Could you check a few things on this model? Use its own coordinates, in mm. Face numbers are marked on the shaded views. A direction names the side the tool comes from. Coordinates: 2 decimals unless noted, no trailing zeros. Order: outer loops, then holes, each group sorted by start corner. A loop starts at its lowest first (then second) coordinate and runs counter-clockwise, first axis right, second up. Notation, with made-up numbers: M -18,55 L 26,55 A16 cw 26,73 Z; hole C -9,78 d2. An arc over 180 degrees is marked long. One line per question, with ' | ' between items. Start each with the question number.
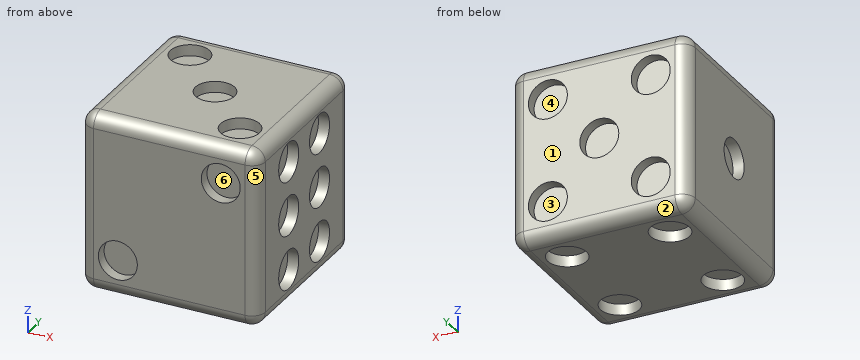
from build123d import *

# Parameters (mm, degrees)
F0_W      = 16
F0_H      = 16
F1_DEPTH  = 16
F2_R      = 1.75
F3_DEPTH  = 1
F4_R      = 1.75
F5_DEPTH  = 1
F6_R      = 1.75
F7_DEPTH  = 1
F8_R      = 1.75
F9_DEPTH  = 1
F10_R     = 1.75
F11_DEPTH = 1
F12_R     = 1.75
F13_DEPTH = 1
F14_R     = 1.2


with BuildPart() as f1:
    # F0 (on Top) → F1 (new body)
    with BuildSketch(Plane.XY):
        Rectangle(F0_W, F0_H)
    extrude(amount=F1_DEPTH)

    # F2 (on face) → F3 (cut)
    with BuildSketch(Plane.XY.offset(16)):
        with Locations((-4.618718, 4.618718)):
            Circle(F2_R)
        with Locations((4.618718, -4.618718)):
            Circle(F2_R)
        Circle(F2_R)
    extrude(amount=-F3_DEPTH, mode=Mode.SUBTRACT)

    # F4 (on face) → F5 (cut)
    with BuildSketch(Plane.XZ.offset(8)):
        with Locations((-4.618718, 3.381282)):
            Circle(F4_R)
        with Locations((4.618718, 12.618718)):
            Circle(F4_R)
    extrude(amount=-F5_DEPTH, mode=Mode.SUBTRACT)

    # F6 (on face) → F7 (cut)
    with BuildSketch(Plane(origin=(-8, 0, 0), x_dir=(0, -1, 0), z_dir=(-1, 0, 0))):
        with Locations((0, 8)):
            Circle(F6_R)
    extrude(amount=-F7_DEPTH, mode=Mode.SUBTRACT)

    # F8 (on face) → F9 (cut)
    with BuildSketch(Plane.YZ.offset(8)):
        with Locations((-2.7, 8)):
            Circle(F8_R)
        with Locations((2.7, 8)):
            Circle(F8_R)
        with Locations((2.7, 12.875)):
            Circle(F8_R)
        with Locations((2.7, 3.125)):
            Circle(F8_R)
        with Locations((-2.7, 3.125)):
            Circle(F8_R)
        with Locations((-2.7, 12.875)):
            Circle(F8_R)
    extrude(amount=-F9_DEPTH, mode=Mode.SUBTRACT)

    # F10 (on face) → F11 (cut)
    with BuildSketch(Plane(origin=(0, 8, 0), x_dir=(-1, 0, 0), z_dir=(0, 1, 0))):
        with Locations((0, 8)):
            Circle(F10_R)
        with Locations((-4.618718, 3.381282)):
            Circle(F10_R)
        with Locations((-4.618718, 12.618718)):
            Circle(F10_R)
        with Locations((4.618718, 12.618718)):
            Circle(F10_R)
        with Locations((4.618718, 3.381282)):
            Circle(F10_R)
    extrude(amount=-F11_DEPTH, mode=Mode.SUBTRACT)

    # F12 (on face) → F13 (cut)
    with BuildSketch(Plane(origin=(0, 0, 0), x_dir=(1, 0, 0), z_dir=(0, 0, -1))):
        with Locations((4.618718, -4.618718)):
            Circle(F12_R)
        with Locations((-4.618718, -4.618718)):
            Circle(F12_R)
        with Locations((-4.618718, 4.618718)):
            Circle(F12_R)
        with Locations((4.618718, 4.618718)):
            Circle(F12_R)
    extrude(amount=-F13_DEPTH, mode=Mode.SUBTRACT)

    # F14
    f14_edges = [f1.edges().sort_by_distance(p)[0] for p in [
        (0, 8, 16),
        (-8, 0, 16),
        (-8, 8, 8),
        (-8, -8, 8),
        (0, -8, 16),
        (8, -8, 8),
        (8, 0, 0),
        (8, 8, 8),
        (0, 8, 0),
        (-8, 0, 0),
        (0, -8, 0),
        (8, 0, 16),
    ]]
    fillet(f14_edges, radius=F14_R)


solid = f1.part
(1) Imagine slicing it at D-D, the plane y = -2. Write out the boundary of the cut face in (x, z).
(2) Imagine slicing it at C-C, the plane x = 0. Write out the boundary of the cut face in (y, z).
(3) On a 3-axis mill with a long thin cutter (end or side, diameter ignored), from which of +Z, -Z, +X, -X, +Y, -Y can I reach the whole of each face in a straight line? I mean the marked faces 4, 5 and 6. Say none if no direction works.
(4) For P1, Ø2, axis at y = 2.7, z = 12.875, coming from the +X side; P2, Ø3, axis at x = 0, y = 0, coming from the +Z side; P3, Ø3, axis at x = -4.5, z = 3.5, coming from the +Y side, each with a flat end and sliding along its axis, tell me the tip position at first contact or that it passes through.
(5) Imagine slicing it at A-A, the plane z = 8. Write out the boundary of the cut face in (x, y), plus the area to 3 significant figures.
(6) Imagine slicing it at B-B, the plane y = 0. Write out the boundary of the cut face in (x, z), plus the area to 3 significant figures.
(7) We'd pull the mould along Z, two halves only. Please class the marked faces 1, 2 and 3: +Z half, -Z half, draft (parallel to the pull), parting line (faces both ways), or undercut.
(8) If I drill on line 1 along Z through (x, y) = (7.65, 2.7) (3 decimals); line 2 along X through (y, z) = (3.25, 1.5); line 3 along Z through (x, y) = (-4.75, 5), over which ranges is the centre line in solid material (lowest first)? Write a range as from..to.
Answers:
1) outline: M -8,1.2 A1.2 ccw -6.8,0 L 6.8,0 A1.2 ccw 8,1.2 L 8,1.52 L 7,1.52 L 7,4.73 L 8,4.73 L 8,6.4 L 7,6.4 L 7,9.6 L 8,9.6 L 8,11.27 L 7,11.27 L 7,14.48 L 8,14.48 L 8,14.8 A1.2 ccw 6.8,16 L -6.8,16 A1.2 ccw -8,14.8 Z
2) outline: M -8,1.2 A1.2 ccw -6.8,0 L 6.8,0 A1.2 ccw 8,1.2 L 8,6.25 L 7,6.25 L 7,9.75 L 8,9.75 L 8,14.8 A1.2 ccw 6.8,16 L 1.75,16 L 1.75,15 L -1.75,15 L -1.75,16 L -6.8,16 A1.2 ccw -8,14.8 Z
3) face 4: +Y | face 5: +Z, -Z, +X, -Y | face 6: -Y
4) P1: x = 7 | P2: z = 15 | P3: y = 7
5) outline: M -8,-6.8 A1.2 ccw -6.8,-8 L 6.8,-8 A1.2 ccw 8,-6.8 L 8,-4.45 L 7,-4.45 L 7,-0.95 L 8,-0.95 L 8,0.95 L 7,0.95 L 7,4.45 L 8,4.45 L 8,6.8 A1.2 ccw 6.8,8 L 1.75,8 L 1.75,7 L -1.75,7 L -1.75,8 L -6.8,8 A1.2 ccw -8,6.8 L -8,1.75 L -7,1.75 L -7,-1.75 L -8,-1.75 Z | area: 241 mm²
6) outline: M -8,1.2 A1.2 ccw -6.8,0 L 6.8,0 A1.2 ccw 8,1.2 L 8,14.8 A1.2 ccw 6.8,16 L 1.75,16 L 1.75,15 L -1.75,15 L -1.75,16 L -6.8,16 A1.2 ccw -8,14.8 L -8,9.75 L -7,9.75 L -7,6.25 L -8,6.25 Z | area: 248 mm²
7) face 1: draft | face 2: -Z half | face 3: undercut
8) line 1: 0.353..1.375, 4.875..6.25, 9.75..11.125, 14.625..15.647 | line 2: -8..7 | line 3: 1..15
